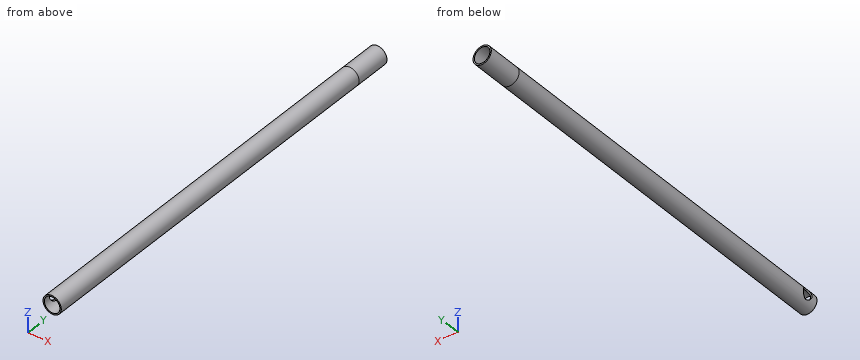
```python
from build123d import *

# Parameters (mm, degrees)
F3_R      = 4.7
F4_DEPTH  = 167
F8_DEPTH  = 167
F6_R      = 4.7
F6_R_2    = 4
F9_DEPTH  = 25
F7_R      = 4.7
F7_R_2    = 4
F10_DEPTH = 18
F11_R     = 2.75
F12_DEPTH = 4.701


# Not quite as in the source:
# - ends of sketch curves that miss each other by under 0.0002 mm in the source are joined


with BuildPart() as f4:
    # F3 (on Front) → F4 (new body)
    with BuildSketch(Plane.XZ):
        Circle(F3_R)
    extrude(amount=F4_DEPTH)

    # F5 (on face) → F8 (cut, through all)
    with BuildSketch(Plane.XZ.offset(167)):
        with BuildLine():
            Line((-1.25, -3.8), (0, -3.8))
            Line((0, -3.8), (1.25, -3.8))
            Line((1.25, -3.8), (1.25, -3.7))
            ThreePointArc((1.25, -3.7), (1.3085786438, -3.5585786438), (1.45, -3.5))
            Line((1.45, -3.5), (2, -3.5))
            Line((2, -3.5), (2, -3.05))
            ThreePointArc((2, -3.05), (2.0585786438, -2.9085786438), (2.2, -2.85))
            Line((2.2, -2.85), (3.15, -2.85))
            Line((3.15, -2.85), (3.15, -2.15))
            Line((3.15, -2.15), (2.2, -2.15))
            ThreePointArc((2.2, -2.15), (2.0585786438, -2.0914213562), (2, -1.95))
            Line((2, -1.95), (2, -1.887459))
            ThreePointArc((2, -1.887459), (2.1033535752, -1.771554046), (2.2, -1.65))
            Line((2.2, -1.65), (3.75, -1.65))
            Line((3.75, -1.65), (3.75, 0))
            Line((3.75, 0), (3.75, 1.65))
            Line((3.75, 1.65), (2.2, 1.65))
            ThreePointArc((2.2, 1.65), (2.1033535752, 1.771554046), (1.9999998047, 1.8874588157))
            Line((1.9999998047, 1.8874588157), (2, 1.95))
            ThreePointArc((2, 1.95), (2.0585786438, 2.0914213562), (2.2, 2.15))
            Line((2.2, 2.15), (3.15, 2.15))
            Line((3.15, 2.15), (3.15, 2.85))
            Line((3.15, 2.85), (2.2, 2.85))
            ThreePointArc((2.2, 2.85), (2.0585786438, 2.9085786438), (2, 3.05))
            Line((2, 3.05), (2, 3.5))
            Line((2, 3.5), (1.45, 3.5))
            ThreePointArc((1.45, 3.5), (1.3085786438, 3.5585786438), (1.25, 3.7))
            Line((1.25, 3.7), (1.25, 3.8))
            Line((1.25, 3.8), (0, 3.8))
            Line((0, 3.8), (-1.25, 3.8))
            Line((-1.25, 3.8), (-1.25, 3.7))
            ThreePointArc((-1.25, 3.7), (-1.3085786438, 3.5585786438), (-1.45, 3.5))
            Line((-1.45, 3.5), (-2, 3.5))
            Line((-2, 3.5), (-2, 3.05))
            ThreePointArc((-2, 3.05), (-2.0585786438, 2.9085786438), (-2.2, 2.85))
            Line((-2.2, 2.85), (-3.15, 2.85))
            Line((-3.15, 2.85), (-3.15, 2.15))
            Line((-3.15, 2.15), (-2.2, 2.15))
            ThreePointArc((-2.2, 2.15), (-2.0585786438, 2.0914213562), (-2, 1.95))
            Line((-2, 1.95), (-2, 1.887459))
            ThreePointArc((-2, 1.887459), (-2.1033535752, 1.771554046), (-2.2, 1.65))
            Line((-2.2, 1.65), (-3.75, 1.65))
            Line((-3.75, 1.65), (-3.75, 0))
            Line((-3.75, 0), (-3.75, -1.65))
            Line((-3.75, -1.65), (-2.2, -1.65))
            ThreePointArc((-2.2, -1.65), (-2.1033535752, -1.771554046), (-1.9999998047, -1.8874588157))
            Line((-1.9999998047, -1.8874588157), (-2, -1.95))
            ThreePointArc((-2, -1.95), (-2.0585786438, -2.0914213562), (-2.2, -2.15))
            Line((-2.2, -2.15), (-3.15, -2.15))
            Line((-3.15, -2.15), (-3.15, -2.85))
            Line((-3.15, -2.85), (-2.2, -2.85))
            ThreePointArc((-2.2, -2.85), (-2.0585786438, -2.9085786438), (-2, -3.05))
            Line((-2, -3.05), (-2, -3.5))
            Line((-2, -3.5), (-1.45, -3.5))
            ThreePointArc((-1.45, -3.5), (-1.3085786438, -3.5585786438), (-1.25, -3.7))
            Line((-1.25, -3.7), (-1.25, -3.8))
        make_face()
    extrude(amount=-F8_DEPTH, mode=Mode.SUBTRACT)

    # F6 (on face) → F9 (join)
    with BuildSketch(Plane.XZ.offset(167)):
        Circle(F6_R)
        Circle(F6_R_2, mode=Mode.SUBTRACT)
    extrude(amount=F9_DEPTH)

    # F7 (on face) → F10 (join)
    with BuildSketch(Plane(origin=(0, 0, 0), x_dir=(-1, 0, 0), z_dir=(0, 1, 0))):
        Circle(F7_R)
        Circle(F7_R_2, mode=Mode.SUBTRACT)
    extrude(amount=F10_DEPTH)

    # F11 (on Right) → F12 (cut, through all)
    with BuildSketch(Plane.YZ):
        with Locations((-186, 0)):
            Circle(F11_R)
    extrude(amount=-F12_DEPTH, mode=Mode.SUBTRACT)


solid = f4.part
```
Design review of the part built by this model. Coordinates are the model's own, in mm. Coordinates: 2 decimals unless noted, no trailing zeros. Order: outer loops, then holes, each group sorted by start corner. A loop starts at its lowest first (then second) coordinate and runs counter-clockwise, first axis right, second up. Notation, with made-up numbers: M 8,32.25 L 62,32.25 A25 cw 62,55.25 Z; hole C 77.5,82 d10. An arc over 180 degrees is marked long. Answer as a JSON object with one key per item and string values. Group by question number.
1) For pin 1 (1 mm diameter, centred on x = 2, z = -0.5, fed in from -Y); pin 2 (0.7 mm diameter, centred on x = -3, z = -2, fed in from +Y); pin 3 (0.5 mm diameter, centred on y = -93.5, z = -3.5, fed in from +X); pin 4 (3 mm diameter, centred on x = -2.5, y = -104, fed in from -Z), all flat-tipped, find the tip position at first contact; note any pin that passes through.
2) Add section A-A, the plane y = -186. Write out the cut boundary in (x, z).
3) Wall thickness on L1, parallel to Z at x = -3, y = -47; L2, parallel to X at y = -106.5, z = 0.5; L3, parallel to X at y = -24, z = -3.75: over which ranges is each line inside the solid? List them lowest first.
Computed values:
{
 "1": {"pin 1": "passes through", "pin 2": "stops at y = 0", "pin 3": "stops at x = 3.4", "pin 4": "stops at z = -4.59"},
 "2": {"outline": "M -3.81,-2.75 A4.7 ccw long -3.81,2.75 L -2.9,2.75 A4 cw long -2.9,-2.75 Z"},
 "3": {"L1": "z = -3.62 to -2.85, -2.15 to -1.65, 1.65 to 2.15, 2.85 to 3.62", "L2": "x = -4.67 to -3.75, 3.75 to 4.67", "L3": "x = -2.83 to -1.25, 1.25 to 2.83"}
}
